Verification items for the finished model (mm, model axes). Face numbers are marked on the shaded views. A direction names the side the tool comes from. Round coordinates to 2 decimals unless told otherwise and drop trailing zeros. Write each loop counter-clockwise with the first axis right and the second up, starting at its lowest first coordinate (ties: lowest second). Pieces come first, ordered by that corner, then holes. Notation, with made-up numbers: M 56,80 L 95,80 A14 ccw 95,94 Z; hole C -38.5,55.25 d6. An arc over 180 degrees is marked long. Use a Markdown table: item, result. Add a question column.
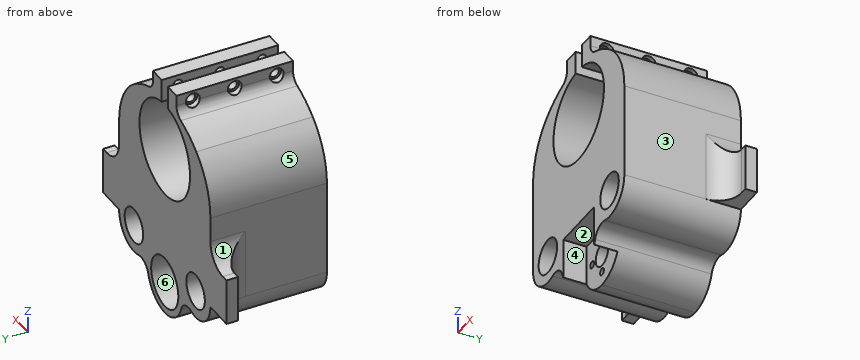
from build123d import *

# Parameters (mm, degrees)
SKETCH1_R           = 7.5
SKETCH1_R_2         = 5.1
BOSS_EXTRUDE1_DEPTH = 50
SKETCH4_R           = 11
CUT_EXTRUDE1_DEPTH  = 15
CUT_EXTRUDE2_REACH  = 97.13
SKETCH5_R           = 1.5
SKETCH7_W           = 25
SKETCH7_H           = 10
CUT_EXTRUDE3_DEPTH  = 25
FILLET1_R           = 25
FILLET2_R           = 25
CUT_EXTRUDE4_REACH  = 107.441
SKETCH9_R           = 2
FILLET3_R           = 5
FILLET4_R           = 5
SKETCH10_R          = 3
CUT_EXTRUDE5_DEPTH  = 2
CUT_EXTRUDE6_DEPTH  = 102.610229819
FILLET5_R           = 30
FILLET6_R           = 30
SKETCH13_W          = 13
SKETCH13_H          = 20
BOSS_EXTRUDE2_DEPTH = 5
FILLET7_R           = 10
FILLET13_R          = 10


with BuildPart() as part:
    # Sketch1 → Boss-Extrude1 (new body)
    with BuildSketch(Plane(origin=(0, 0, 0), x_dir=(1, 0, 0), z_dir=(0, 1, 0))):
        with BuildLine():
            Line((2.5, -70.346989949), (2.5, -80.346989949))
            Line((2.5, -80.346989949), (9.5, -80.346989949))
            Line((9.5, -80.346989949), (9.5, -72))
            ThreePointArc((9.5, -72), (25.801442039, -64.189302549), (37, -50))
            Line((37, -50), (37, 25))
            Line((37, 25), (-37, 25))
            Line((-37, 25), (-37, -50))
            ThreePointArc((-37, -50), (-25.801442039, -64.189302549), (-9.5, -72))
            Line((-9.5, -72), (-9.5, -80.346989949))
            Line((-9.5, -80.346989949), (-2.5, -80.346989949))
            Line((-2.5, -80.346989949), (-2.5, -70.346989949))
            ThreePointArc((-2.5, -70.346989949), (0, -29.5), (2.5, -70.346989949))
        make_face()
        with Locations(Location((25, 0, 0), (0, 0, 270))):
            Circle(SKETCH1_R, mode=Mode.SUBTRACT)
        with Locations(Location((-25, 0, 0), (0, 0, 270))):
            Circle(SKETCH1_R, mode=Mode.SUBTRACT)
        with Locations(Location((0, 11, 0), (0, 0, 270))):
            Circle(SKETCH1_R_2, mode=Mode.SUBTRACT)
    extrude(amount=BOSS_EXTRUDE1_DEPTH)

    # Sketch4 → Cut-Extrude1 (cut)
    with BuildSketch(Plane(origin=(0, 50, 0), x_dir=(1, 0, 0), z_dir=(0, 1, 0))):
        with Locations(Location((0, 11, 0), (0, 0, 270))):
            Circle(SKETCH4_R)
    extrude(amount=-CUT_EXTRUDE1_DEPTH, mode=Mode.SUBTRACT)

    # Sketch5 → Cut-Extrude2 (cut, up to next)
    with BuildSketch(Plane(origin=(0, 35, 0), x_dir=(1, 0, 0), z_dir=(0, 1, 0)), mode=Mode.PRIVATE) as cut_extrude2_sk1:
        with Locations(Location((0, 19, 0), (0, 0, 270))):
            Circle(SKETCH5_R)
    cut_extrude2_tool1 = extrude(cut_extrude2_sk1.sketch, amount=-CUT_EXTRUDE2_REACH, mode=Mode.PRIVATE) & part.part
    # Sketch5 → Cut-Extrude2 (cut, up to next)
    with BuildSketch(Plane(origin=(0, 35, 0), x_dir=(1, 0, 0), z_dir=(0, 1, 0)), mode=Mode.PRIVATE) as cut_extrude2_sk2:
        with Locations(Location((8, 11, 0), (0, 0, 270))):
            Circle(SKETCH5_R)
    cut_extrude2_tool2 = extrude(cut_extrude2_sk2.sketch, amount=-CUT_EXTRUDE2_REACH, mode=Mode.PRIVATE) & part.part
    # Sketch5 → Cut-Extrude2 (cut, up to next)
    with BuildSketch(Plane(origin=(0, 35, 0), x_dir=(1, 0, 0), z_dir=(0, 1, 0)), mode=Mode.PRIVATE) as cut_extrude2_sk3:
        with Locations(Location((0, 3, 0), (0, 0, 270))):
            Circle(SKETCH5_R)
    cut_extrude2_tool3 = extrude(cut_extrude2_sk3.sketch, amount=-CUT_EXTRUDE2_REACH, mode=Mode.PRIVATE) & part.part
    # Sketch5 → Cut-Extrude2 (cut, up to next)
    with BuildSketch(Plane(origin=(0, 35, 0), x_dir=(1, 0, 0), z_dir=(0, 1, 0)), mode=Mode.PRIVATE) as cut_extrude2_sk4:
        with Locations(Location((-8, 11, 0), (0, 0, 270))):
            Circle(SKETCH5_R)
    cut_extrude2_tool4 = extrude(cut_extrude2_sk4.sketch, amount=-CUT_EXTRUDE2_REACH, mode=Mode.PRIVATE) & part.part
    add(cut_extrude2_tool1.solids().sort_by_distance((0, 35, -19))[0], mode=Mode.SUBTRACT)
    add(cut_extrude2_tool2.solids().sort_by_distance((8, 35, -11))[0], mode=Mode.SUBTRACT)
    add(cut_extrude2_tool3.solids().sort_by_distance((0, 35, -3))[0], mode=Mode.SUBTRACT)
    add(cut_extrude2_tool4.solids().sort_by_distance((-8, 35, -11))[0], mode=Mode.SUBTRACT)

    # Sketch7 → Cut-Extrude3 (cut)
    with BuildSketch(Plane(origin=(0, 0, -25), x_dir=(-1, 0, 0), z_dir=(0, 0, -1))):
        with Locations((0, 5)):
            Rectangle(SKETCH7_W, SKETCH7_H)
    extrude(amount=-CUT_EXTRUDE3_DEPTH, mode=Mode.SUBTRACT)

    # Fillet1
    fillet1_edges = [part.edges().sort_by_distance(p)[0] for p in [
        (37, 25, -25),
    ]]
    fillet(fillet1_edges, radius=FILLET1_R)

    # Fillet2
    fillet2_edges = [part.edges().sort_by_distance(p)[0] for p in [
        (-37, 25, -25),
    ]]
    fillet(fillet2_edges, radius=FILLET2_R)

    # Cut-Extrude4: up to this face of the body (flat: up to its plane)
    cut_extrude4_end = Plane(part.part.faces().sort_by_distance((9.5, 25, 76.173494975))[0])
    # Sketch9 → Cut-Extrude4 (cut, up to the picked face)
    with BuildSketch(Plane.ZY.offset(9.5), mode=Mode.PRIVATE) as cut_extrude4_sk1:
        with Locations((76.173494975, 43)):
            Circle(SKETCH9_R)
    cut_extrude4_tool1 = split(extrude(cut_extrude4_sk1.sketch, amount=-CUT_EXTRUDE4_REACH, mode=Mode.PRIVATE), bisect_by=cut_extrude4_end, keep=Keep.BOTH, mode=Mode.PRIVATE)
    # Sketch9 → Cut-Extrude4 (cut, up to the picked face)
    with BuildSketch(Plane.ZY.offset(9.5), mode=Mode.PRIVATE) as cut_extrude4_sk2:
        with Locations((76.173494975, 7)):
            Circle(SKETCH9_R)
    cut_extrude4_tool2 = split(extrude(cut_extrude4_sk2.sketch, amount=-CUT_EXTRUDE4_REACH, mode=Mode.PRIVATE), bisect_by=cut_extrude4_end, keep=Keep.BOTH, mode=Mode.PRIVATE)
    # Sketch9 → Cut-Extrude4 (cut, up to the picked face)
    with BuildSketch(Plane.ZY.offset(9.5), mode=Mode.PRIVATE) as cut_extrude4_sk3:
        with Locations((76.173494975, 25)):
            Circle(SKETCH9_R)
    cut_extrude4_tool3 = split(extrude(cut_extrude4_sk3.sketch, amount=-CUT_EXTRUDE4_REACH, mode=Mode.PRIVATE), bisect_by=cut_extrude4_end, keep=Keep.BOTH, mode=Mode.PRIVATE)
    add(cut_extrude4_tool1.solids().sort_by(Axis((-9.5, 43, 76.173495), (1, 0, 0)))[0], mode=Mode.SUBTRACT)
    add(cut_extrude4_tool2.solids().sort_by(Axis((-9.5, 7, 76.173495), (1, 0, 0)))[0], mode=Mode.SUBTRACT)
    add(cut_extrude4_tool3.solids().sort_by(Axis((-9.5, 25, 76.173495), (1, 0, 0)))[0], mode=Mode.SUBTRACT)

    # Fillet3
    # the kernel refuses this fillet: 5 mm, written as the material it adds along each edge
    with BuildSketch(Plane(origin=(-9.5, 0, 72), x_dir=(-0.9653617561408162, 0, -0.2609150815509128), z_dir=(0, 1, 0))) as fillet3_piece_1_section:
        with BuildLine():
            CenterArc((3.829392618, 4.994923289), FILLET3_R, 195.124366766, 72.293488253)
            Line((-0.997416163, 3.690347881), (0, 0))
            ThreePointArc((0, 0), (1.802067114, 0.040613692), (3.604134229, 0))
        make_face()
    fillet3_piece_1 = extrude(amount=50, mode=Mode.PRIVATE)
    fillet3_piece_1 = fillet3_piece_1 - Plane(origin=(-10.278685319, 43, 76.173494975), x_dir=(0, 0, 1), z_dir=(-1, 0, 0)) * Cylinder(2, 115, mode=Mode.PRIVATE)
    fillet3_piece_1 = fillet3_piece_1 - Plane(origin=(-10.278685319, 25, 76.173494975), x_dir=(0, 0, 1), z_dir=(-1, 0, 0)) * Cylinder(2, 115, mode=Mode.PRIVATE)
    fillet3_piece_1 = fillet3_piece_1 - Plane(origin=(-10.278685319, 7, 76.173494975), x_dir=(0, 0, 1), z_dir=(-1, 0, 0)) * Cylinder(2, 115, mode=Mode.PRIVATE)
    add(fillet3_piece_1)

    # Fillet4
    # the kernel refuses this fillet: 5 mm, written as the material it adds along each edge
    with BuildSketch(Plane(origin=(9.5, 0, 72), x_dir=(0.9653617561408171, 0, -0.2609150815509095), z_dir=(0, 1, 0))) as fillet4_piece_1_section:
        with BuildLine():
            CenterArc((3.829392618, -4.994923289), FILLET4_R, 92.582144981, 72.293488253)
            Line((-0.997416163, -3.690347881), (0, 0))
            ThreePointArc((0, 0), (1.802067114, -0.040613692), (3.604134229, 0))
        make_face()
    fillet4_piece_1 = extrude(amount=50, mode=Mode.PRIVATE)
    fillet4_piece_1 = fillet4_piece_1 - Plane(origin=(10.278685319, 43, 76.173494975), x_dir=(0, 0, 1), z_dir=(-1, 0, 0)) * Cylinder(2, 115, mode=Mode.PRIVATE)
    fillet4_piece_1 = fillet4_piece_1 - Plane(origin=(10.278685319, 25, 76.173494975), x_dir=(0, 0, 1), z_dir=(-1, 0, 0)) * Cylinder(2, 115, mode=Mode.PRIVATE)
    fillet4_piece_1 = fillet4_piece_1 - Plane(origin=(10.278685319, 7, 76.173494975), x_dir=(0, 0, 1), z_dir=(-1, 0, 0)) * Cylinder(2, 115, mode=Mode.PRIVATE)
    add(fillet4_piece_1)

    # Sketch10 → Cut-Extrude5 (cut, symmetric)
    with BuildSketch(Plane.ZY.offset(9.5)):
        with Locations(Location((76.173494975, 7, 0), (0, 0, 96.713867574))):
            Circle(SKETCH10_R)
        with Locations(Location((76.173494975, 43, 0), (0, 0, 180))):
            Circle(SKETCH10_R)
        with Locations(Location((76.173494975, 25, 0), (0, 0, 96.713867574))):
            Circle(SKETCH10_R)
    cut_extrude5 = extrude(amount=CUT_EXTRUDE5_DEPTH, both=True, mode=Mode.SUBTRACT)

    # Mirror1: Cut-Extrude5 across plane
    add(cut_extrude5.mirror(Plane(origin=(0, 0, 0), x_dir=(0, 0, 1), z_dir=(1, 0, 0))), mode=Mode.SUBTRACT)

    # Sketch11 → Cut-Extrude6 (cut, through all)
    with BuildSketch(Plane(origin=(0, 50, 0), x_dir=(1, 0, 0), z_dir=(0, 1, 0))):
        with BuildLine():
            ThreePointArc((37, 0), (29.67766953, 17.67766953), (12, 25))
            Line((12, 25), (0, 25))
            ThreePointArc((0, 25), (8.213758719, 22.337291022), (13.303110425, 15.362023959))
            ThreePointArc((13.303110425, 15.362023959), (16.428719044, 11.73096472), (21.207236508, 11.384855954))
            ThreePointArc((21.207236508, 11.384855954), (32.017365535, 9.734299202), (37, 0))
        make_face()
        with BuildLine():
            ThreePointArc((-13.303110425, 15.362023959), (-8.213758719, 22.337291022), (0, 25))
            Line((0, 25), (-12, 25))
            ThreePointArc((-12, 25), (-29.67766953, 17.67766953), (-37, 0))
            ThreePointArc((-37, 0), (-32.017365535, 9.734299202), (-21.207236508, 11.384855954))
            ThreePointArc((-21.207236508, 11.384855954), (-16.428719044, 11.73096472), (-13.303110425, 15.362023959))
        make_face()
    extrude(amount=-CUT_EXTRUDE6_DEPTH, mode=Mode.SUBTRACT)

    # Fillet5
    fillet5_edges = [part.edges().sort_by_distance(p)[0] for p in [
        (-37, 25, 50),
    ]]
    fillet(fillet5_edges, radius=FILLET5_R)

    # Fillet6
    fillet6_edges = [part.edges().sort_by_distance(p)[0] for p in [
        (37, 25, 50),
    ]]
    fillet(fillet6_edges, radius=FILLET6_R)

    # Sketch13 → Boss-Extrude2 (add)
    with BuildSketch(Plane(origin=(0, 50, 0), x_dir=(1, 0, 0), z_dir=(0, 1, 0))):
        with Locations((43.5, -10)):
            Rectangle(SKETCH13_W, SKETCH13_H)
    boss_extrude2 = extrude(amount=-BOSS_EXTRUDE2_DEPTH)

    # Mirror2: Boss-Extrude2 across plane
    add(boss_extrude2.mirror(Plane(origin=(0, 0, 0), x_dir=(0, 0, 1), z_dir=(1, 0, 0))))

    # Fillet7
    fillet7_edges = [part.edges().sort_by_distance(p)[0] for p in [
        (37, 45, 10),
        (37, 47.5, 20),
    ]]
    fillet(fillet7_edges, radius=FILLET7_R)

    # Fillet13
    fillet13_edges = [part.edges().sort_by_distance(p)[0] for p in [
        (-37, 47.5, 20),
        (-37, 45, 10),
    ]]
    fillet(fillet13_edges, radius=FILLET13_R)


solid = part.part
1. Depth check by flat-ended pin: pin 1 Ø2.5 at (x, z) = (48.5, 6.5) entering from -Y; pin 2 Ø8 at (y, z) = (42, 44) entering from -X; pin 3 Ø4 at (y, z) = (25.5, 16) entering from +X. Enter the tip coordinate at first touch or a pass-through.
2. Cross-section at A-A on x = 16. Enter the section's corners in (y, z), plus the area to 3 significant figures.
3. Cross-section at C-C on y = 32. Enter the section's corners in (x, z), plus the area to 3 significant figures.
4. Release check for a two-part mould opening along X. For the marked faces 1, 2 and 3 record: +X half, -X half, draft (parallel to the pull), parting line (faces both ways), or undercut.
5. Access from +Z, -Z, +X, -X, +Y, -Y to the whole of each face (thin tool, end or side, straight path). Record for the marked faces 4, 5 and 6.
6. Cross-section at B-B on z = 33. Enter the section's corners in (x, y), plus the area to 3 significant figures.
7. Scan lines: line 1 along X through (y, z) = (28.5, 0); line 2 along Z through (x, y) = (8.9, 7); line 3 along Z through (x, y) = (-8.5, 8). Record each from-to range of solid material in increasing order. Write a range as from..to.
8. Cross-section at D-D on z = -3. Enter the section's corners in (x, y).
Answer:
| question | item | result |
|---|---|---|
| 1 | pin 1 | stops at y = 45 |
| 1 | pin 2 | stops at x = -37 |
| 1 | pin 3 | stops at x = 37 |
| 2 | outline | M 0,-11.97 L 50,-11.97 L 50,37.18 L 0,37.18 Z; M 0,62.82 L 50,62.82 L 50,69.96 L 0,69.96 Z |
| 2 | area | 2,810 mm^2 |
| 3 | outline | M -37,0 A12 ccw -21.21,-11.38 A6.24 cw -13.3,-15.36 A14 ccw 13.3,-15.36 A6.24 cw 21.21,-11.38 A12 ccw 37,0 L 37,40.81 A30 ccw 25.56,64.38 A40 ccw 12.98,71.06 A5 cw 9.5,75.82 L 9.5,80.35 L 2.5,80.35 L 2.5,70.35 A20.5 cw long -2.5,70.35 L -2.5,80.35 L -9.5,80.35 L -9.5,75.82 A5 cw -12.98,71.06 A40 ccw -25.56,64.38 A30 ccw -37,40.81 Z; hole C -25,0 d15; hole C -8,-11 d3; hole C 0,-11 d10.2; hole C 0,-19 d3; hole C 0,-3 d3; hole C 8,-11 d3; hole C 25,0 d15 |
| 3 | area | 4,320 mm^2 |
| 4 | face 1 | -X half |
| 4 | face 2 | undercut |
| 4 | face 3 | +X half |
| 5 | face 4 | -Z, -Y |
| 5 | face 5 | +Z, -X, +Y, -Y |
| 5 | face 6 | +Y |
| 6 | outline | M -37,0 L -11.46,0 L -11.46,50 L -37,50 Z; M 11.46,0 L 37,0 L 37,50 L 11.46,50 Z |
| 6 | area | 2,550 mm^2 |
| 7 | line 1 | x = -37..-32.5, -17.5..17.5, 32.5..37 |
| 7 | line 2 | z = 0..31.53, 68.47..73.17, 79.17..80.35 |
| 7 | line 3 | z = 0..31.35, 68.65..73.35, 79..80.35 |
| 8 | outline | M -36.62,0 L -31.87,0 L -31.87,50 L -36.62,50 Z; M -18.13,0 L -12.5,0 L -12.5,10 L -1.5,10 L -1.5,35 L -7.55,35 L -7.55,50 L -18.13,50 Z; M 1.5,10 L 12.5,10 L 12.5,0 L 18.13,0 L 18.13,50 L 7.55,50 L 7.55,35 L 1.5,35 Z; M 31.87,0 L 36.62,0 L 36.62,50 L 31.87,50 Z |
